Read the model definition and answer for the solid it produces. Units are mm, in the model's axes. Coordinates: 2 decimals unless noted, no trailing zeros. Loops run counter-clockwise (first coordinate to the right, second up) from the corner with the lowest first, then second, coordinate; pieces in that order, holes last. Notation, with made-up numbers: M 41.5,45 L 57.5,45 A18 ccw 57.5,62 Z; hole C 18.25,30 d7. An arc over 180 degrees is marked long. Use one line per item in the form item = value. Start each with the question number.
1. Flat-ended cylindrical pins translate along their axes: pin 1 (0.7 mm diameter, centred on y = -17, z = 1789.5, fed in from +X); pin 2 (2.5 mm diameter, centred on y = -11, z = 1146.5, fed in from +X); pin 3 (0.7 mm diameter, centred on y = -17, z = 1513, fed in from -X). Find the tip coordinate at first contact, or state that the pin passes through.
2. The part is cut by section A-A (z = 1190). Give the vertices of the cut face in (x, y).
3. Find the intervals of material crossed by probe 1 along X at (y, z) = (-16.25, 301); probe 2 along X at (y, z) = (-14.25, 2042); probe 3 along Y at (x, z) = (11, 320), in increasing order. Write a range as [from, to].
from build123d import *

# Parameters (mm, degrees)
ESTRUSIONE_ESTRUSIONE1_DEPTH = 2897


with BuildPart() as part:
    # Schizzo1 → Estrusione-Estrusione1 (new body)
    with BuildSketch(Plane.XY):
        with BuildLine():
            Line((-10.087089482, -16.415981983), (-7.565622613, -13.894515114))
            Line((-7.565622613, -13.894515114), (-7.565622613, -8.851581376))
            Line((-7.565622613, -8.851581376), (-8.0775657, -8.339638289))
            ThreePointArc((-8.0775657, -8.339638289), (-8.808436534, -6.752953221), (-10.395121602, -6.022082387))
            Line((-10.395121602, -6.022082387), (-10.591382856, -5.825821133))
            Line((-10.591382856, -5.825821133), (-10.591382856, -2.800060891))
            Line((-10.591382856, -2.800060891), (-10.395121602, -2.603799637))
            ThreePointArc((-10.395121602, -2.603799637), (-8.808436534, -1.872928803), (-8.0775657, -0.286243735))
            Line((-8.0775657, -0.286243735), (-7.565622613, 0.225699352))
            Line((-7.565622613, 0.225699352), (9.580352097, 0.225699352))
            Line((9.580352097, 0.225699352), (10.092295184, -0.286243735))
            ThreePointArc((10.092295184, -0.286243735), (10.823166018, -1.872928803), (12.409851086, -2.603799637))
            Line((12.409851086, -2.603799637), (12.606112339, -2.800060891))
            Line((12.606112339, -2.800060891), (12.606112339, -5.825821133))
            Line((12.606112339, -5.825821133), (12.409851086, -6.022082387))
            ThreePointArc((12.409851086, -6.022082387), (10.823166018, -6.752953221), (10.092295184, -8.339638289))
            Line((10.092295184, -8.339638289), (9.580352097, -8.851581376))
            Line((9.580352097, -8.851581376), (9.580352097, -13.894515114))
            Line((9.580352097, -13.894515114), (12.101818966, -16.415981983))
            Line((12.101818966, -16.415981983), (12.101818966, -17.774300648))
            Line((12.101818966, -17.774300648), (-10.087089482, -17.774300648))
            Line((-10.087089482, -17.774300648), (-10.087089482, -16.415981983))
        make_face()
    extrude(amount=ESTRUSIONE_ESTRUSIONE1_DEPTH)


solid = part.part
Computed values:
q1.pin_1 = 12.1
q1.pin_2 = 9.58
q1.pin_3 = -10.09
q2.outline = M -10.59,-5.83 L -10.4,-6.02 A2.52 cw -8.08,-8.34 L -7.57,-8.85 L -7.57,-13.89 L -10.09,-16.42 L -10.09,-17.77 L 12.1,-17.77 L 12.1,-16.42 L 9.58,-13.89 L 9.58,-8.85 L 10.09,-8.34 A2.52 cw 12.41,-6.02 L 12.61,-5.83 L 12.61,-2.8 L 12.41,-2.6 A2.52 cw 10.09,-0.29 L 9.58,0.23 L -7.57,0.23 L -8.08,-0.29 A2.52 cw -10.4,-2.6 L -10.59,-2.8 Z
q3.probe_1 = [-9.92, 11.94]
q3.probe_2 = [-7.92, 9.94]
q3.probe_3 = [-17.77, -15.31], [-6.59, -2.03]
